Geometry check sheet. Reference: the model listing, model coordinates, mm. Face numbers are marked on the shaded views. Round coordinates to 2 decimals unless told otherwise and drop trailing zeros. Loops run counter-clockwise (first coordinate to the right, second up) from the corner with the lowest first, then second, coordinate; pieces in that order, holes last. Notation, with made-up numbers: (-20.75, 87.25) - (13.25, 87.25) arc R13 ccw to (13.25, 94.25) - close; hole circle Ø3 at (-5.5, 11). An arc over 180 degrees is marked (long way). Answer as CSV lines item,"result". Start each with the question number.
1) Cross-section at A-A on z = 0. Record the boundary of the cut face in (x, y), and give its area (3 significant figures).
2) Cross-section at D-D on x = 0.5. Record the boundary of the cut face in (y, z), and give its area (3 significant figures).
3) Draft check along Z on the marked faces 1, 2, 3 and 4. Enter one of: released by +Z, released by -Z, zero draft, split by the parting line, or undercut.
4) Depth check by flat-ended pin: P1, Ø1, axis at y = -7, z = 4.5, coming from the +X side; P2, Ø4, axis at y = 1, z = -3.5, coming from the +X side. Enter the tip coordinate at first touch or a pass-through.
5) Cross-section at C-C on x = -4. Record the boundary of the cut face in (y, z), and give its area (3 significant figures).
6) Thickness scan on line 1 along X through (y, z) = (-4.25, 2.75); line 2 along Z through (x, y) = (0, 6.25); line 3 along X through (y, z) = (-1, 3.25). Record the ranges inside material, lowest first.
from build123d import *

# Parameters (mm, degrees)
F1_DEPTH = 11
F2_R     = 0.99999


# Not quite as in the source:
# - a fillet or chamfer is up to 0.001 mm smaller than in the source, because OpenCascade refuses the exact size


with BuildPart() as f1:
    # F0 (on Front) → F1 (new body, symmetric)
    with BuildSketch(Plane.XZ):
        with BuildLine():
            Line((-3.5, -6.0621778265), (-2.5, -4.3301270189))
            ThreePointArc((-2.5, -4.3301270189), (-2.5, 4.3301270189), (5, 0))
            ThreePointArc((5, 0), (4.3301270189, -2.5), (2.5, -4.3301270189))
            Line((2.5, -4.3301270189), (3.5, -6.0621778265))
            ThreePointArc((3.5, -6.0621778265), (6.0621778265, -3.5), (7, 0))
            ThreePointArc((7, 0), (-3.5, 6.0621778265), (-3.5, -6.0621778265))
        make_face()
    extrude(amount=F1_DEPTH, both=True)

    # F2 (radius 1 in the source; OpenCascade refuses exactly that, so slightly less here)
    f2_edges = [f1.edges().sort_by_distance(p)[0] for p in [
        (3.5, 5.5, -6.062178),
        (3.5, -5.5, -6.062178),
        (2.5, -5.5, -4.330127),
        (-2.5, -5.5, -4.330127),
        (-3.5, 5.5, -6.062178),
        (-3.5, -5.5, -6.062178),
    ]]
    fillet(f2_edges, radius=F2_R)


solid = f1.part
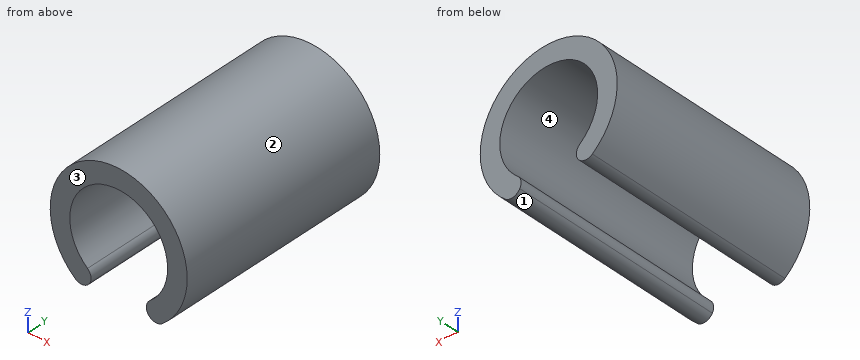
Answer block:
1,outline,"(-7, -11) - (-5, -11) - (-5, 11) - (-7, 11) - close; (5, -11) - (7, -11) - (7, 11) - (5, 11) - close"
1,area,"88.0 mm^2"
2,outline,"(-11, 4.97) - (11, 4.97) - (11, 6.98) - (-11, 6.98) - close"
2,area,"44.2 mm^2"
3,face 1,"released by -Z"
3,face 2,"split by the parting line"
3,face 3,"zero draft"
3,face 4,"undercut"
4,P1,"stops at x = 5.74"
4,P2,"stops at x = 6.84"
5,outline,"(-11, -5.61) - (11, -5.61) - (11, -3) - (-11, -3) - close; (-11, 3) - (11, 3) - (11, 5.74) - (-11, 5.74) - close"
5,area,"118 mm^2"
6,line 1,"x = -6.44 to -4.18, 4.18 to 6.44"
6,line 2,"z = 5 to 7"
6,line 3,"x = -6.2 to -3.8, 3.8 to 6.2"
